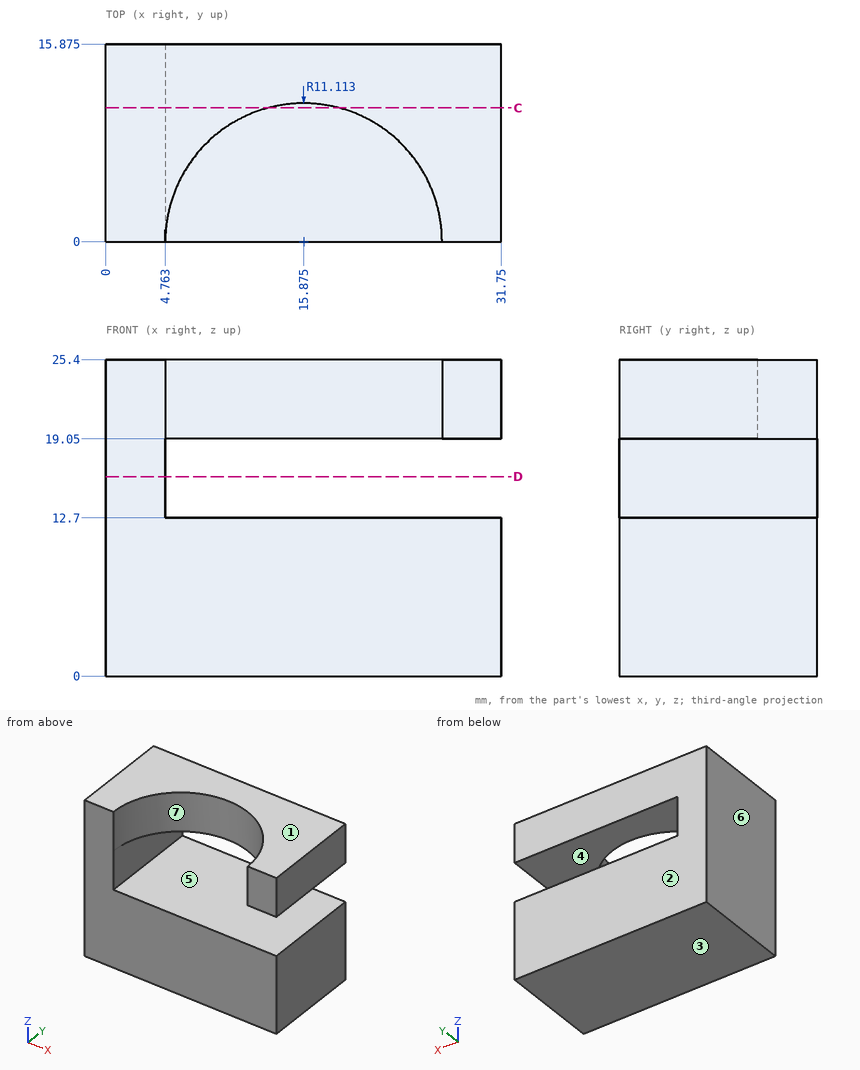
For this review, use the dimensioned drawing (mm, ordinates from the lowest corner) and the shaded views. A direction names the side the tool comes from. Coordinates: 2 decimals unless noted, no trailing zeros. Order: outer loops, then holes, each group sorted by start corner. A loop starts at its lowest first (then second) coordinate and runs counter-clockwise, first axis right, second up. Notation, with made-up numbers: (39, 58) - (59, 58) arc R19 cw to (59, 88) - close; hole circle Ø2 at (13, -3.75). An arc over 180 degrees is marked (long way). Use one line per item in the form item = value.
Q1. For probe 1 along Z at (x, y) = (26.5, 11.5); probe 2 along X at (y, z) = (7.75, 23.5); probe 3 along Z at (x, y) = (22, 8.5), list the stretches that pass through material, from the lowest coordinate up. Write a range as from..to.
Checked values:
probe_1 = 0..12.7, 19.05..25.4
probe_2 = 0..7.91, 23.84..31.75
probe_3 = 0..12.7
Q2. Consider section D-D (z = 16). Give the boundary of the cut face in (x, y) (1 decimal).
Checked values:
outline = (0, 0) - (4.8, 0) - (4.8, 15.9) - (0, 15.9) - close
Q3. For P1, Ø3, axis at y = 9.5, z = 15.5, coming from the +X side, flat-tipped, find the tip position at first contact; note if it passes through.
Checked values:
P1 = 4.76
Q4. Consider section C-C (y = 10.75). Give the boundary of the cut face in (x, z).
Checked values:
outline = (0, 0) - (31.75, 0) - (31.75, 12.7) - (4.76, 12.7) - (4.76, 19.05) - (13.06, 19.05) - (13.06, 25.4) - (0, 25.4) - close; (18.69, 19.05) - (31.75, 19.05) - (31.75, 25.4) - (18.69, 25.4) - close
Q5. Draft analysis for pull direction Z (two halves, no side actions). For the marked faces 1, 2, 3 and 4, state which applies: +Z half, -Z half, draft (parallel to the pull), parting line (faces both ways), or undercut.
Checked values:
face_1 = +Z half
face_2 = draft
face_3 = -Z half
face_4 = undercut
Q6. For the marked faces 5, 6 and 7, list the 3-axis set-ups (+Z, -Z, +X, -X, +Y, -Y) from which the entire face can be reached by the end or side of a thin tool; tool diameter is ignored.
Checked values:
face_5 = +X, +Y, -Y
face_6 = +Z, -Z, -X, +Y, -Y
face_7 = +Z, -Y
